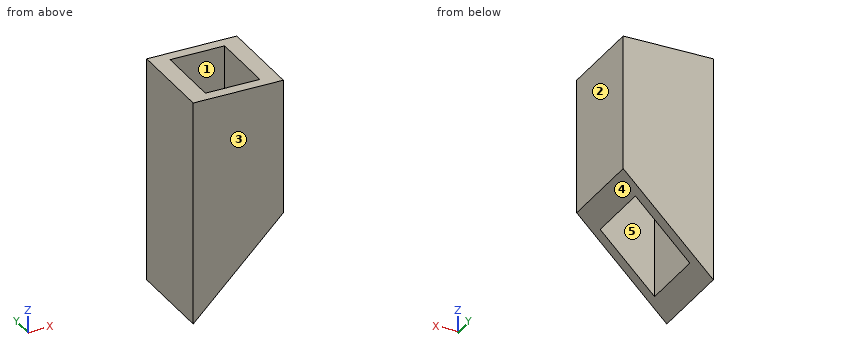
```python
from build123d import *

# Parameters (mm, degrees)
F0_W      = 50.8
F0_H      = 50.8
F0_W_2    = 47.625
F0_H_2    = 47.625
F1_DEPTH  = 508
F3_DEPTH  = 50.801
F5_DEPTH  = 50.801
F7_W      = 101.6
F7_H      = 101.6
F7_W_2    = 61.3725754684
F7_H_2    = 76.9944727293
F8_DEPTH  = 254
F10_DEPTH = 101.601


with BuildPart() as f1:
    # F0 (on Top) → F1 (new body)
    with BuildSketch(Plane.XY):
        Rectangle(F0_W, F0_H)
        Rectangle(F0_W_2, F0_H_2, mode=Mode.SUBTRACT)
    extrude(amount=F1_DEPTH)

    # F2 (on face) → F3 (cut, through all)
    with BuildSketch(Plane.XZ.offset(25.4)):
        Polygon((25.4, 46.0020601749), (-25.4, 0), (25.4, 0), align=None)
    extrude(amount=-F3_DEPTH, mode=Mode.SUBTRACT)

    # F4 (on face) → F5 (cut, through all)
    with BuildSketch(Plane.XZ.offset(25.4)):
        Polygon((25.4, 508), (-25.4, 508), (25.4, 469.4332480431), align=None)
    extrude(amount=-F5_DEPTH, mode=Mode.SUBTRACT)


with BuildPart() as f8:
    # F7 (on Top) → F8 (new body)
    with BuildSketch(Plane.XY):
        Rectangle(F7_W, F7_H)
        Rectangle(F7_W_2, F7_H_2, mode=Mode.SUBTRACT)
    extrude(amount=F8_DEPTH)

    # F9 (on face) → F10 (cut, through all)
    with BuildSketch(Plane.XZ.offset(50.8)):
        Polygon((50.8, 101.6), (-50.8, 0), (50.8, 0), align=None)
    extrude(amount=-F10_DEPTH, mode=Mode.SUBTRACT)


solid = f8.part
```
Input: part model. Units: mm. Frame: model coordinates. Face numbers are marked on the shaded views. A direction names the side the tool comes from. Round coordinates to 2 decimals unless told otherwise and drop trailing zeros. Loops run counter-clockwise (first coordinate to the right, second up) from the corner with the lowest first, then second, coordinate; pieces in that order, holes last.
1) Pin query (flat end, axial travel): pin 1 (1.5 mm diameter, centred on x = 37, y = 37.5, fed in from -Z); pin 2 (10 mm diameter, centred on y = -0.5, z = 90, fed in from +X). Return the tip coordinate at first contact, or that it passes through.
Ans:
pin 1: stops at z = 87.05
pin 2: stops at x = 44.2
2) Section query B-B on z = 91. Return the cut outline in (x, y).
Ans:
outline: (-50.8, -50.8) - (40.2, -50.8) - (40.2, 50.8) - (-50.8, 50.8) - close; hole (-30.69, -38.5) - (30.69, -38.5) - (30.69, 38.5) - (-30.69, 38.5) - close
3) Section query C-C on y = -3. Return the cut outline in (x, z).
Ans:
outline: (-50.8, 0) - (-30.69, 20.11) - (-30.69, 254) - (-50.8, 254) - close; (30.69, 81.49) - (50.8, 101.6) - (50.8, 254) - (30.69, 254) - close
4) Material intervals for line 1 (X direction, y = 1.5, z = 227.5); line 2 (Y direction, x = -17.5, z = 230); line 3 (X direction, y = -13.5, z = 92), sorted ascending.
Ans:
line 1: x = -50.8 to -30.69, 30.69 to 50.8
line 2: y = -50.8 to -38.5, 38.5 to 50.8
line 3: x = -50.8 to -30.69, 30.69 to 41.2
5) Set-up query: the marked faces 4 and 5. Return all of +Z, -Z, +X, -X, +Y, -Y with unobstructed straight access to the full face (end or side cutting, diameter ignored); none if empty.
Ans:
face 4: -Z, +X, +Y, -Y
face 5: +Z, -Z
6) Section query D-D on z = 63. Return the cut outline in (x, y), plus the area to 3 significant figures.
Ans:
outline: (-50.8, -50.8) - (12.2, -50.8) - (12.2, -38.5) - (-30.69, -38.5) - (-30.69, 38.5) - (12.2, 38.5) - (12.2, 50.8) - (-50.8, 50.8) - close
area: 3,100 mm2
7) Section query A-A on x = 15.5. Return the cut outline in (y, z), plus the area to 3 significant figures.
Ans:
outline: (-50.8, 66.3) - (-38.5, 66.3) - (-38.5, 254) - (-50.8, 254) - close; (38.5, 66.3) - (50.8, 66.3) - (50.8, 254) - (38.5, 254) - close
area: 4,620 mm2
8) Pull-direction query (Y, two-part tool) for the marked faces 1, 2 and 3; classes: released by +Y, released by -Y, zero draft, split by the parting line, or undercut.
Ans:
face 1: undercut
face 2: zero draft
face 3: released by -Y
